CAD build for the part. Positions are in the model's coordinates, mm. Face numbers are marked on the shaded views. Round coordinates to 2 decimals unless told otherwise and drop trailing zeros. Write each loop counter-clockwise with the first axis right and the second up, starting at its lowest first coordinate (ties: lowest second). Pieces come first, ordered by that corner, then holes. Notation, with made-up numbers: (-14, 14) - (-1, 14) arc R23 ccw to (-1, 24) - close; hole circle Ø3 at (-32.75, 22.25). An arc over 180 degrees is marked (long way). Answer in a Markdown table with one row per item.
```python
from build123d import *

# Parameters (mm, degrees)
BOSS_EXTRUDE1_DEPTH    = 3.175
CUT_EXTRUDE1_DEPTH     = 3.175
F_10_CLEARANCE_HOLE1_D = 5.1054
FILLET1_R              = 6.35
FILLET2_R              = 2.54
F_10_CLEARANCE_HOLE2_D = 5.1054
FILLET3_DEPTH          = 3.175
FILLET4_DEPTH          = 3.175


with BuildPart() as part:
    # Sketch1 → Boss-Extrude1 (new body)
    with BuildSketch(Plane.XY):
        Polygon((0, 0), (-203.2, 0), (-203.2, 22.225), (16.492698582, 74.393755743), (150.197623574, -38.509278075), (138.121306744, -64.407023089), align=None)
    extrude(amount=BOSS_EXTRUDE1_DEPTH)

    # Sketch2 → Cut-Extrude1 (cut)
    with BuildSketch(Plane.XY.offset(3.175)):
        with BuildLine():
            ThreePointArc((21.24883588, 4.583754924), (18.61914073, 2.941077903), (15.535547838, 3.265329747))
            Line((15.535547838, 3.265329747), (126.332322757, -48.400054896))
            Line((126.332322757, -48.400054896), (80.920020655, 3.146145486))
            Line((80.920020655, 3.146145486), (21.24883588, 4.583754924))
        make_face()
        with BuildLine():
            Line((137.027076007, -44.215538399), (138.486158755, -41.086525347))
            Line((138.486158755, -41.086525347), (98.909290031, -7.667049227))
            Line((98.909290031, -7.667049227), (129.564314023, -42.462686891))
            ThreePointArc((129.564314023, -42.462686891), (133.738335549, -41.454571408), (137.027076007, -44.215538399))
        make_face()
        Polygon((-0.44732738, 12.687080727), (10.590747216, 63.202397136), (-71.622854337, 43.679757896), align=None)
        Polygon((-76.769135969, 38.994763822), (-144.447250959, 9.525), (-9.091020978, 9.525), align=None)
        Polygon((-94.260732486, 38.304112991), (-152.4, 24.498222921), (-152.4, 12.98794568), align=None)
        with BuildLine():
            Line((78.512994475, 9.555978624), (16.762189587, 61.699556828))
            Line((16.762189587, 61.699556828), (5.751368588, 11.308965438))
            Line((5.751368588, 11.308965438), (14.340754941, 11.102028322))
            ThreePointArc((14.340754941, 11.102028322), (17.662973074, 12.342739027), (20.921588597, 10.943481637))
            Line((20.921588597, 10.943481637), (78.512994475, 9.555978624))
        make_face()
    extrude(amount=-CUT_EXTRUDE1_DEPTH, mode=Mode.SUBTRACT)

    # #10 Clearance Hole1 (through all)
    with Locations(Plane.XY.offset(3.175)):
        with Locations((15.118307034, 68.194276097), (1.099513239, 4.959583716), (90.351919236, 2.887547679), (-83.537983118, 43.502605356)):
            Hole(F_10_CLEARANCE_HOLE1_D / 2)

    # Fillet1
    fillet1_edges = [part.edges().sort_by_distance(p)[0] for p in [
        (0, 0, 1.5875),
        (16.492698582, 74.393755743, 1.5875),
    ]]
    fillet(fillet1_edges, radius=FILLET1_R)

    # Fillet2
    fillet2_edges = [part.edges().sort_by_distance(p)[0] for p in [
        (80.920020655, 3.146145486, 1.5875),
        (126.332322757, -48.400054896, 1.5875),
        (20.921588597, 10.943481637, 1.5875),
        (14.340754941, 11.102028322, 1.5875),
        (5.751368588, 11.308965438, 1.5875),
        (16.762189587, 61.699556828, 1.5875),
        (-0.44732738, 12.687080727, 1.5875),
        (-71.622854337, 43.679757896, 1.5875),
        (10.590747216, 63.202397136, 1.5875),
        (-94.260732486, 38.304112991, 1.5875),
        (-152.4, 12.98794568, 1.5875),
        (-152.4, 24.498222921, 1.5875),
        (129.564314023, -42.462686891, 1.5875),
        (98.909290031, -7.667049227, 1.5875),
        (-76.769135969, 38.994763822, 1.5875),
        (-9.091020978, 9.525, 1.5875),
        (-144.447250959, 9.525, 1.5875),
    ]]
    fillet(fillet2_edges, radius=FILLET2_R)

    # #10 Clearance Hole2 (through all)
    with Locations(Plane.XY.offset(3.175)):
        with Locations((17.54826731, 7.581620583), (132.649356264, -46.090898658)):
            Hole(F_10_CLEARANCE_HOLE2_D / 2)

    # Fillet3: read off the stored shape, not the designer's step
    # Fillet3 outline → Fillet3 (add)
    with BuildSketch(Plane.XY):
        with BuildLine():
            Line((15.535547838, 3.265329747), (21.232159568, 0.608956072))
            add(Edge.make_bspline(
                [(21.232159568, 0.608956072), (19.885857145, 1.236747202), (19.378566273, 2.827814172), (20.725192465, 4.03358552)],
                knots=[0, 0, 0, 0, 0.69383671, 0.69383671, 0.69383671, 0.69383671], degree=3, weights=[1, 0.632112013, 0.519478217, 0.662098611]))
            ThreePointArc((20.725192465, 4.03358552), (18.245689672, 2.870462732), (15.535547838, 3.265329747))
        make_face()
        with BuildLine():
            ThreePointArc((21.24883588, 4.583754924), (20.997999412, 4.298214627), (20.725192465, 4.03358552))
            add(Edge.make_bspline(
                [(20.725192465, 4.03358552), (21.150941215, 4.414801664), (21.664082636, 4.573750721), (22.158575797, 4.561837299)],
                knots=[0.69383671, 0.69383671, 0.69383671, 0.69383671, 1, 1, 1, 1], degree=3, weights=[0.662098611, 0.725031472, 0.837665268, 1]))
            Line((22.158575797, 4.561837299), (21.24883588, 4.583754924))
        make_face()
    extrude(amount=FILLET3_DEPTH)

    # Fillet4: read off the stored shape, not the designer's step
    # Fillet4 outline → Fillet4 (add)
    with BuildSketch(Plane.XY):
        with BuildLine():
            Line((138.486158755, -41.086525347), (137.659679105, -40.38862989))
            add(Edge.make_bspline(
                [(137.659679105, -40.38862989), (137.885417825, -40.579248046), (138.092627638, -40.854150437), (138.228700196, -41.219427367), (138.224361363, -41.647951666), (138.029002465, -42.066900176)],
                knots=[0, 0, 0, 0, 0, 0, 0.431143376, 0.431143376, 0.431143376, 0.431143376, 0.431143376, 0.431143376], degree=5, weights=[1, 0.825460303, 0.688546423, 0.58925836, 0.527596114, 0.503559686]))
            Line((138.029002465, -42.066900176), (138.486158755, -41.086525347))
        make_face()
        with BuildLine():
            Line((137.027076007, -44.215538399), (138.029002465, -42.066900176))
            add(Edge.make_bspline(
                [(138.029002465, -42.066900176), (137.740787916, -42.684978272), (137.186504044, -43.023143687), (136.590787826, -43.018448848), (136.121756233, -42.804773213), (135.808946692, -42.527417975)],
                knots=[0.431143376, 0.431143376, 0.431143376, 0.431143376, 0.431143376, 0.431143376, 1, 1, 1, 1, 1, 1], degree=5, weights=[0.503559686, 0.471845684, 0.505632715, 0.604920778, 0.769709873, 1]))
            ThreePointArc((135.808946692, -42.527417975), (136.511376305, -43.304107052), (137.027076007, -44.215538399))
        make_face()
    extrude(amount=FILLET4_DEPTH)


solid = part.part
```
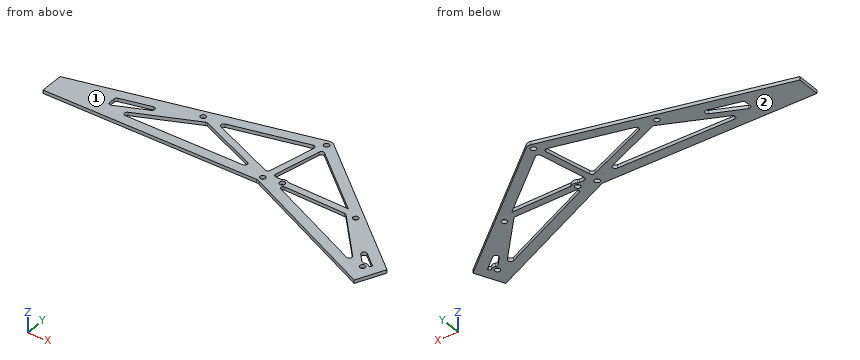
Q1. Saw through at D-D on x = 67. List the corners of the cut face in (y, z) (1 decimal).
Computed:
| item | result |
|---|---|
| outline | (-31.2, 0) - (-20.7, 0) - (-20.7, 3.2) - (-31.2, 3.2) - close; (3.5, 0) - (9.8, 0) - (9.8, 3.2) - (3.5, 3.2) - close; (19.3, 0) - (31.7, 0) - (31.7, 3.2) - (19.3, 3.2) - close |
Q2. Saw through at C-C on z = 0.85. Count the separate pieces of the cut face and the enclosed holes in it, then the cut area to 3 significant figures.
Computed:
| item | result |
|---|---|
| separate pieces | 1 |
| enclosed holes | 12 |
| area | 10,200 mm2 |
Q3. Saw through at A-A on y = -7. List the corners of the cut face in (x, z) (3 decimals), then the cut area to 3 significant figures.
Computed:
| item | result |
|---|---|
| outline | (15.012, 0) - (37.55, 0) - (37.55, 3.175) - (15.012, 3.175) - close; (89.859, 0) - (112.883, 0) - (112.883, 3.175) - (89.859, 3.175) - close |
| area | 145 mm2 |
Q4. Pull direction Z, two halves, no side cores. Call the marked faces 1 and 2: released by +Z, released by -Z, zero draft, split by the parting line, or undercut.
Computed:
| item | result |
|---|---|
| face 1 | released by +Z |
| face 2 | released by -Z |
Q5. Saw through at B-B on x = -125.5. List the corners of the cut face in (y, z) (3 decimals), then the cut area to 3 significant figures.
Computed:
| item | result |
|---|---|
| outline | (0, 0) - (9.525, 0) - (9.525, 3.175) - (0, 3.175) - close; (17.775, 0) - (24.701, 0) - (24.701, 3.175) - (17.775, 3.175) - close; (30.886, 0) - (40.676, 0) - (40.676, 3.175) - (30.886, 3.175) - close |
| area | 83.3 mm2 |
Q6. Flat gauge pins, fed straight in: pin 1 (3 mm diameter, centred on x = -130.5, y = 20, fed in from -Z); pin 2 (4 mm diameter, centred on x = 17.55, y = 7.58, fed in from -Z). Where does each tip first touch, or does it go through?
Computed:
| item | result |
|---|---|
| pin 1 | stops at z = 0 |
| pin 2 | passes through |
Q7. Drill centre lines: line 1 (Y direction, x = -120, z = 1.7) (3 decimals); line 2 (Y direction, x = 76, z = 0.7); line 3 (X direction, y = -40, z = 2.05). Where is each one in solid material? Low to high.
Computed:
| item | result |
|---|---|
| line 1 | y = 0 to 9.525, 20.17 to 27.147, 31.331 to 41.982 |
| line 2 | y = -35.44 to -24.93, 3.26 to 9.62, 11.68 to 24.14 |
| line 3 | x = 85.78 to 108.32, 118.75 to 127.39, 137.2 to 149.5 |
